from build123d import *

# Parameters (mm, degrees)
BOSS_EXTRUDE1_DEPTH      = 31.75
X_0_397_DIAMETER_HOLE1_D = 10.795
CHAMFER1_SIZE            = 1.27
CHAMFER2_SIZE            = 0.254
FILLET1_R                = 0.254


with BuildPart() as part:
    # Sketch1 → Boss-Extrude1 (new body)
    with BuildSketch(Plane.XY):
        with BuildLine():
            Line((46.736, 0), (46.736, 17.145))
            Line((46.736, 17.145), (20.193, 17.145))
            Line((20.193, 17.145), (20.193, 27.94))
            Line((20.193, 27.94), (0, 27.94))
            Line((0, 27.94), (0, 26.67))
            ThreePointArc((0, 26.67), (12.7, 13.97), (0, 1.27))
            Line((0, 1.27), (0, 0))
            Line((0, 0), (46.736, 0))
        make_face()
    extrude(amount=BOSS_EXTRUDE1_DEPTH)

    # X (0.397) Diameter Hole1 (through all)
    with Locations(Plane(origin=(0, 17.145, 0), x_dir=(1, 0, 0), z_dir=(0, 1, 0))):
        with Locations((33.02, -15.875)):
            Hole(X_0_397_DIAMETER_HOLE1_D / 2)

    # Chamfer1
    chamfer1_edges = [part.edges().sort_by_distance(p)[0] for p in [
        (46.736, 17.145, 15.875),
    ]]
    chamfer(chamfer1_edges, length=CHAMFER1_SIZE)

    # Chamfer2
    chamfer2_edges = [part.edges().sort_by_distance(p)[0] for p in [
        (38.4175, 17.145, 15.875),
    ]]
    chamfer(chamfer2_edges, length=CHAMFER2_SIZE)

    # Fillet1
    fillet1_edges = [part.edges().sort_by_distance(p)[0] for p in [
        (20.193, 17.145, 15.875),
    ]]
    fillet(fillet1_edges, radius=FILLET1_R)


solid = part.part
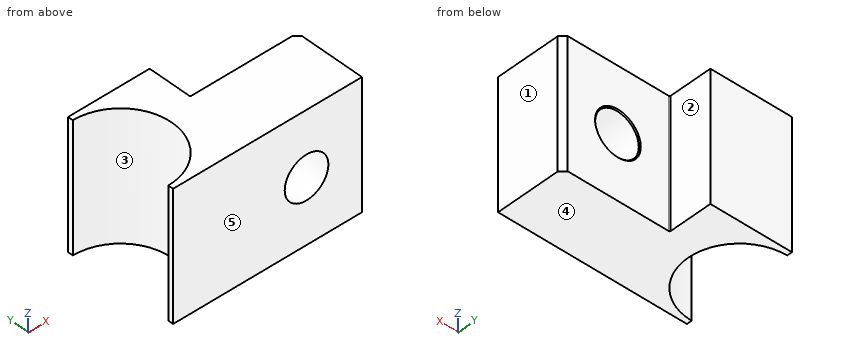
Input: part model. Units: mm. Frame: model coordinates. Face numbers are marked on the shaded views. A direction names the side the tool comes from. Round coordinates to 2 decimals unless told otherwise and drop trailing zeros. Loops run counter-clockwise (first coordinate to the right, second up) from the corner with the lowest first, then second, coordinate; pieces in that order, holes last. Notation, with made-up numbers: (40, 37) -> (46, 37) arc R17 cw to (46, 45) -> close; hole circle Ø5 at (-5, -6.75). An arc over 180 degrees is marked (long way). Answer as a JSON object with one key per item and string values. Group by question number.
1) Ray query, L1, parallel to Z at x = 33.02, y = 6.75; L2, parallel to Y at x = 5, z = 22.5; L3, parallel to Y at x = 40.5, z = 7 (3 decimals). Return the intervals inside material, ascending.
2) Section query C-C on z = 26.5. Output: boundary loops of the cut face in (x, y) (3 decimals).
3) Section query D-D on x = 9. Output: boundary loops of the cut face in (y, z), plus the area to 3 significant figures.
4) Reachability of the marked faces 1 and 2 from +Z, -Z, +X, -X, +Y, -Y: full face, straight path, thin tool, end or side. Return the list, or none.
5) Draft query along Y for the marked faces 3, 4 and 5. Return one class per face: +Y half, -Y half, draft (parallel to the pull), parting line (faces both ways), or undercut.
6) Pin query (flat end, axial travel): pin 1 (5 mm diameter, centred on x = 29, z = 20, fed in from +Y) (3 decimals); pin 2 (1.5 mm diameter, centred on y = 3, z = 12.5, fed in from -X). Return the tip coordinate at first contact, or that it passes through.
Reply:
{
 "1": {"L1": "z = 0 to 10.48, 21.27 to 31.75", "L2": "y = 0 to 2.3, 25.64 to 27.94", "L3": "y = 0 to 17.145"},
 "2": {"outline": "(0, 0) -> (46.736, 0) -> (46.736, 15.875) -> (45.466, 17.145) -> (20.447, 17.145) arc R0.254 cw to (20.193, 17.399) -> (20.193, 27.94) -> (0, 27.94) -> (0, 26.67) arc R12.7 cw to (0, 1.27) -> close"},
 "3": {"outline": "(0, 0) -> (5.01, 0) -> (5.01, 31.75) -> (0, 31.75) -> close; (22.93, 0) -> (27.94, 0) -> (27.94, 31.75) -> (22.93, 31.75) -> close", "area": "318 mm2"},
 "4": {"face 1": "+Z, -Z, +X, +Y, -Y", "face 2": "+Z, -Z, +X, +Y"},
 "5": {"face 3": "undercut", "face 4": "draft", "face 5": "-Y half"},
 "6": {"pin 1": "stops at y = 17.145", "pin 2": "stops at x = 4.89"}
}
